Model file for the job. Use its own axes, mm. Face numbers are marked on the shaded views. A direction names the side the tool comes from. Coordinates: 2 decimals unless noted, no trailing zeros. Write each loop counter-clockwise with the first axis right and the second up, starting at its lowest first coordinate (ties: lowest second). Pieces come first, ordered by that corner, then holes.
Q1. Pull direction Z, two halves, no side cores. Call the marked faces 1, 2, 3 and 4: released by +Z, released by -Z, zero draft, split by the parting line, or undercut.
Q2. Which spindle directions (+Z, -Z, +X, -X, +Y, -Y) get a long thin tool onto all of the face, cutting with end or side? Do the marked faces 5 and 6. Say none if no direction does.
Q3. Band-saw the part on C-C, the plane z = -11. Write the cut outline in (x, y).
Q4. Band-saw the part on A-A, the plane x = 64.5. Write the cut outline in (y, z).
Q5. Band-saw the part on B-B, the plane y = 3.5. State how many separate pieces and enclosed holes the cut face has, plus the area to 3 significant figures.
Q6. Drill centre lines: probe 1 along Z at (x, y) = (68, 6.25); probe 2 along X at (y, z) = (1, -13.75); probe 3 along X at (y, z) = (4.75, -7.75). Where is each one in solid material? Low to high.
from build123d import *

# Parameters (mm, degrees)
SKETCH1_W           = 78
SKETCH1_H           = 20
BOSS_EXTRUDE1_DEPTH = 6.5
SKETCH2_R           = 2.5
CUT_EXTRUDE1_DEPTH  = 81.785209042
SKETCH3_W           = 15
SKETCH3_H           = 6.5
CUT_EXTRUDE2_DEPTH  = 81.785209042
FILLET1_R           = 10


with BuildPart() as part:
    # Sketch1 → Boss-Extrude1 (new body)
    with BuildSketch(Plane(origin=(0, 0, 0), x_dir=(1, 0, 0), z_dir=(0, 1, 0))):
        with Locations((39, 10)):
            Rectangle(SKETCH1_W, SKETCH1_H)
    extrude(amount=BOSS_EXTRUDE1_DEPTH)

    # Sketch2 → Cut-Extrude1 (cut, through all)
    with BuildSketch(Plane(origin=(0, 6.5, 0), x_dir=(1, 0, 0), z_dir=(0, 1, 0))):
        with Locations(Location((10, 10, 0), (0, 0, 270))):
            Circle(SKETCH2_R)
    extrude(amount=-CUT_EXTRUDE1_DEPTH, mode=Mode.SUBTRACT)

    # Sketch3 → Cut-Extrude2 (cut, through all)
    with BuildSketch(Plane(origin=(0, 6.5, 0), x_dir=(1, 0, 0), z_dir=(0, 1, 0))):
        with Locations((64, 13.25)):
            Rectangle(SKETCH3_W, SKETCH3_H)
    extrude(amount=-CUT_EXTRUDE2_DEPTH, mode=Mode.SUBTRACT)

    # Fillet1
    fillet1_edges = [part.edges().sort_by_distance(p)[0] for p in [
        (0, 3.25, 0),
        (0, 3.25, -20),
    ]]
    fillet(fillet1_edges, radius=FILLET1_R - 0.0001)  # a hair under: the kernel refuses the full size


solid = part.part
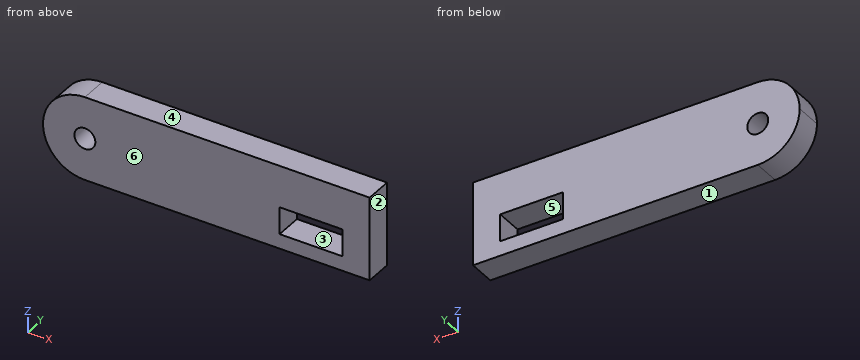
Answer sheet:
1. face 1: released by -Z
1. face 2: zero draft
1. face 3: undercut
1. face 4: released by +Z
2. face 5: +Y, -Y
2. face 6: +Z, -Z, +X, -X, -Y
3. outline: (0.05, 0) - (7.71, 0) - (7.71, 6.5) - (0.05, 6.5) - close; (12.29, 0) - (56.5, 0) - (56.5, 6.5) - (12.29, 6.5) - close; (71.5, 0) - (78, 0) - (78, 6.5) - (71.5, 6.5) - close
4. outline: (0, -20) - (6.5, -20) - (6.5, -16.5) - (0, -16.5) - close; (0, -10) - (6.5, -10) - (6.5, 0) - (0, 0) - close
5. separate pieces: 1
5. enclosed holes: 2
5. area: 1,400 mm2
6. probe 1: z = -20 to -16.5, -10 to 0
6. probe 2: x = 0.73 to 56.5, 71.5 to 78
6. probe 3: x = 0.26 to 8.91, 11.09 to 78
